from build123d import *

# Parameters (mm, degrees)
CYLINDER009_R     = 4
CYLINDER009_DEPTH = 4
CYLINDER011_R     = 4
CYLINDER011_DEPTH = 4
CYLINDER010_R     = 4
CYLINDER010_DEPTH = 4
CYLINDER012_R     = 4
CYLINDER012_DEPTH = 4
CYLINDER007_R     = 2
CYLINDER007_DEPTH = 17
CYLINDER005_R     = 2
CYLINDER005_DEPTH = 17
CYLINDER006_R     = 2
CYLINDER006_DEPTH = 17
CYLINDER008_R     = 2
CYLINDER008_DEPTH = 17
CYLINDER004_R     = 4
CYLINDER004_DEPTH = 10
CYLINDER003_R     = 4
CYLINDER003_DEPTH = 10
CYLINDER002_R     = 4
CYLINDER002_DEPTH = 10
CYLINDER001_R     = 4
CYLINDER001_DEPTH = 10
CYLINDER_R        = 45
CYLINDER_DEPTH    = 15
FILLET001_R       = 0.1
BOX_W             = 92
BOX_H             = 92
BOX_DEPTH         = 12
FILLET_R          = 0.3


with BuildPart() as cylinder009:
    # Cylinder009 → Cylinder009 (new body)
    with BuildSketch(Plane(origin=(41.25, 41.25, 10), x_dir=(1, 0, 0), z_dir=(0, 0, 1))):
        Circle(CYLINDER009_R)
    extrude(amount=CYLINDER009_DEPTH)


with BuildPart() as cylinder011:
    # Cylinder011 → Cylinder011 (new body)
    with BuildSketch(Plane(origin=(-41.25, -41.25, 10), x_dir=(1, 0, 0), z_dir=(0, 0, 1))):
        Circle(CYLINDER011_R)
    extrude(amount=CYLINDER011_DEPTH)


with BuildPart() as cylinder010:
    # Cylinder010 → Cylinder010 (new body)
    with BuildSketch(Plane(origin=(-41.25, 41.25, 10), x_dir=(1, 0, 0), z_dir=(0, 0, 1))):
        Circle(CYLINDER010_R)
    extrude(amount=CYLINDER010_DEPTH)


with BuildPart() as fusion004:
    # Cylinder012 → Cylinder012 (new body)
    with BuildSketch(Plane(origin=(41.25, -41.25, 10), x_dir=(1, 0, 0), z_dir=(0, 0, 1))):
        Circle(CYLINDER012_R)
    extrude(amount=CYLINDER012_DEPTH)

    # Fusion004: union Cylinder009, Cylinder011, Cylinder010
    add(cylinder009.part)
    add(cylinder011.part)
    add(cylinder010.part)


with BuildPart() as cylinder007:
    # Cylinder007 → Cylinder007 (new body)
    with BuildSketch(Plane(origin=(41.25, -41.25, -3), x_dir=(1, 0, 0), z_dir=(0, 0, 1))):
        Circle(CYLINDER007_R)
    extrude(amount=CYLINDER007_DEPTH)


with BuildPart() as cylinder005:
    # Cylinder005 → Cylinder005 (new body)
    with BuildSketch(Plane(origin=(41.25, 41.25, -3), x_dir=(1, 0, 0), z_dir=(0, 0, 1))):
        Circle(CYLINDER005_R)
    extrude(amount=CYLINDER005_DEPTH)


with BuildPart() as cylinder006:
    # Cylinder006 → Cylinder006 (new body)
    with BuildSketch(Plane(origin=(-41.25, 41.25, -3), x_dir=(1, 0, 0), z_dir=(0, 0, 1))):
        Circle(CYLINDER006_R)
    extrude(amount=CYLINDER006_DEPTH)


with BuildPart() as fusion003:
    # Cylinder008 → Cylinder008 (new body)
    with BuildSketch(Plane(origin=(-41.25, -41.25, -3), x_dir=(1, 0, 0), z_dir=(0, 0, 1))):
        Circle(CYLINDER008_R)
    extrude(amount=CYLINDER008_DEPTH)

    # Fusion003: union Cylinder007, Cylinder005, Cylinder006
    add(cylinder007.part)
    add(cylinder005.part)
    add(cylinder006.part)


with BuildPart() as cylinder004:
    # Cylinder004 → Cylinder004 (new body)
    with BuildSketch(Plane(origin=(-41.25, -41.25, 0), x_dir=(1, 0, 0), z_dir=(0, 0, 1))):
        Circle(CYLINDER004_R)
    extrude(amount=CYLINDER004_DEPTH)


with BuildPart() as cylinder003:
    # Cylinder003 → Cylinder003 (new body)
    with BuildSketch(Plane(origin=(41.25, -41.25, 0), x_dir=(1, 0, 0), z_dir=(0, 0, 1))):
        Circle(CYLINDER003_R)
    extrude(amount=CYLINDER003_DEPTH)


with BuildPart() as cylinder002:
    # Cylinder002 → Cylinder002 (new body)
    with BuildSketch(Plane(origin=(-41.25, 41.25, 0), x_dir=(1, 0, 0), z_dir=(0, 0, 1))):
        Circle(CYLINDER002_R)
    extrude(amount=CYLINDER002_DEPTH)


with BuildPart() as cylinder001:
    # Cylinder001 → Cylinder001 (new body)
    with BuildSketch(Plane(origin=(41.25, 41.25, 0), x_dir=(1, 0, 0), z_dir=(0, 0, 1))):
        Circle(CYLINDER001_R)
    extrude(amount=CYLINDER001_DEPTH)


with BuildPart() as cone001:
    # Cone001 → Cone001 (revolve)
    with BuildSketch(Plane(origin=(0, 0, 2), x_dir=(1, 0, 0), z_dir=(0, -1, 0))):
        Polygon((0, 0), (45, 0), (65.25, 12), (0, 12), align=None)
    revolve(axis=Axis((0, 0, 2), (0, 0, 1)))


with BuildPart() as void:
    # Cylinder → Cylinder (new body)
    with BuildSketch(Plane.XY.offset(-1)):
        Circle(CYLINDER_R)
    extrude(amount=CYLINDER_DEPTH)

    # Fusion001: union Cone001
    add(cone001.part)


with BuildPart() as fillet001:
    # Cone → Cone (revolve)
    with BuildSketch(Plane.XZ):
        Polygon((0, 0), (45, 0), (65.25, 12), (0, 12), align=None)
    revolve(axis=Axis((0, 0, 0), (0, 0, 1)))

    # Fillet001
    fillet001_edges = [fillet001.edges().sort_by_distance(p)[0] for p in [
        (-65.25, 0, 12),
    ]]
    fillet(fillet001_edges, radius=FILLET001_R)


with BuildPart() as cut002:
    # Box → Box (new body)
    with BuildSketch(Plane(origin=(-46, -46, 0), x_dir=(1, 0, 0), z_dir=(0, 0, 1))):
        with Locations((46, 46)):
            Rectangle(BOX_W, BOX_H)
    extrude(amount=BOX_DEPTH)

    # Fillet
    fillet_edges = [cut002.edges().sort_by_distance(p)[0] for p in [
        (-46, -46, 6),
        (-46, 46, 6),
        (-46, 0, 0),
        (46, -46, 6),
        (46, 46, 6),
        (46, 0, 0),
        (0, -46, 0),
        (0, 46, 0),
    ]]
    fillet(fillet_edges, radius=FILLET_R)

    # Fusion: union Fillet001
    add(fillet001.part)

    # Cut: cut void
    add(void.part, mode=Mode.SUBTRACT)

    # Fusion002: union Cylinder004, Cylinder003, Cylinder002, Cylinder001
    add(cylinder004.part)
    add(cylinder003.part)
    add(cylinder002.part)
    add(cylinder001.part)

    # Cut001: cut Fusion003
    add(fusion003.part, mode=Mode.SUBTRACT)

    # Cut002: cut Fusion004
    add(fusion004.part, mode=Mode.SUBTRACT)


solid = cut002.part
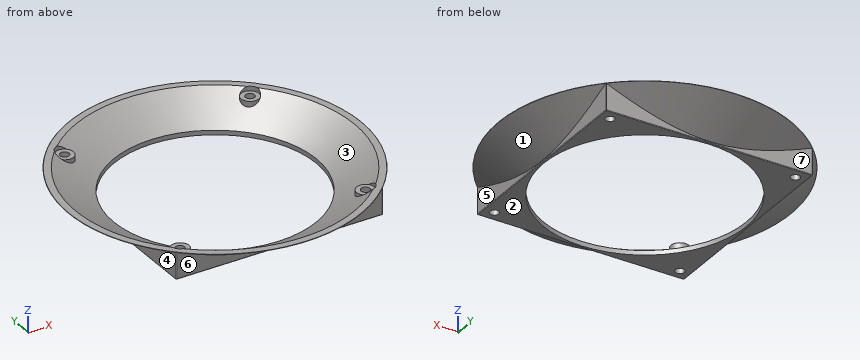
Could you check a few things on this model? Use its own coordinates, in mm. Face numbers are marked on the shaded views. A direction names the side the tool comes from. Coordinates: 2 decimals unless noted, no trailing zeros. Write each loop counter-clockwise with the first axis right and the second up, starting at its lowest first coordinate (ties: lowest second). Pieces come first, ordered by that corner, then holes. Notation, with made-up numbers: (27.5, -32) - (66.5, -32) arc R26 ccw to (66.5, 6) - close; hole circle Ø11 at (68.5, -10.75). An arc over 180 degrees is marked (long way). Put each result on its own line as item: value. Start each with the question number.
Q1. I'm going to push flat-ended pins straight in: P1, Ø6, axis at y = -39.5, z = 10, coming from the +X side; P2, Ø5, axis at x = 41.25, y = 41.25, coming from the +Z side; P3, Ø3.5, axis at x = -10, z = 9, coming from the +Y side; P4, Ø2.5, axis at x = -41.25, y = 41.25, coming from the -Z side. Where does each tip first touch, or does it pass through?
Q2. Which directions (+Z, -Z, +X, -X, +Y, -Y) give clear straight access to the entire face, cutting with the end or side of a thin tool? Please do the marked faces 4, 5, 6 and 7.
Q3. Please list where these lines run through material, in increasing order: L1, parallel to X at y = 0, z = 0.45; L2, parallel to X at y = 21.5, z = 2.25; L3, parallel to Y at x = 0, z = 0.65.
Q4. I want a section at B-B on y = 0. Write out the boundary of the cut face in (x, z) (3 decimals).
Q5. I want a section at C-C on z = 6. Write out the boundary of the cut face in (x, y) (3 decimals), plus the area to 3 significant figures.
Q6. Thinking about a two-plate mould opening in X: for the marked faces 1, 2 and 3, which applies, pulls with the +X half, pulls with the -X half, needs draft (parallel to the pull), parting line crosses it, or undercut?
Checks:
1. P1: x = 53.31
1. P2: z = 10
1. P3: y = 62.36
1. P4: through
2. face 4: -Z, -X
2. face 5: -Z, +X
2. face 6: -Z, -Y
2. face 7: -Z, +Y
3. L1: -46 to -45, 45 to 46
3. L2: -46 to -40.01, 40.01 to 46
3. L3: -46.1 to -45, 45 to 46.1
4. outline: (-64.936, 11.814) - (-46, 0.593) - (-46, 0.3) arc R0.3 ccw to (-45.7, 0) - (-45, 0) - (-45, 2) - (-61.875, 12) - (-64.885, 12) arc R0.1 ccw to start; (45, 0) - (45.7, 0) arc R0.3 ccw to (46, 0.3) - (46, 0.593) - (64.936, 11.814) arc R0.1 ccw to (64.885, 12) - (61.875, 12) - (45, 2) - close
5. outline: (-46, -45.7) arc R0.3 ccw to (-45.7, -46) - (-30.377, -46) arc R55.125 ccw to (30.377, -46) - (45.7, -46) arc R0.3 ccw to (46, -45.7) - (46, -30.377) arc R55.125 ccw to (46, 30.377) - (46, 45.7) arc R0.3 ccw to (45.7, 46) - (30.377, 46) arc R55.125 ccw to (-30.377, 46) - (-45.7, 46) arc R0.3 ccw to (-46, 45.7) - (-46, 30.377) arc R55.125 ccw to (-46, -30.377) - close; hole circle Ø103.5 at (0, 0); hole circle Ø4 at (-41.25, -41.25); hole circle Ø4 at (-41.25, 41.25); hole circle Ø4 at (41.25, -41.25); hole circle Ø4 at (41.25, 41.25)
5. area: 1,500 mm²
6. face 1: parting line crosses it
6. face 2: needs draft
6. face 3: undercut
